```python
from build123d import *

# Parameters (mm, degrees)
SKETCH_1_W          = 26
SKETCH_1_H          = 16
EXTRUDE_1_DEPTH     = 2
EXTRUDE_2_DEPTH     = 2
FILLET_1_R          = 5
FILLET_2_R          = 3
SKETCH_4_R          = 4
CUT_EXTRUDE_1_DEPTH = 38.312866414
SKETCH_5_R          = 2.15
CUT_EXTRUDE_2_DEPTH = 34.648922717
FILLET_3_R          = 3
FILLET_START        = -13
FILLET_4_DEPTH      = 26.69955789
FILLET_START_2      = 4
FILLET_4_2_DEPTH    = 2


with BuildPart() as part:
    # 草图1 → 凸台-拉伸1 (new body)
    with BuildSketch(Plane(origin=(0, 0, 0), x_dir=(1, 0, 0), z_dir=(0, 1, 0))):
        Rectangle(SKETCH_1_W, SKETCH_1_H)
    extrude(amount=EXTRUDE_1_DEPTH)

    # 草图3 → 凸台-拉伸2 (add)
    with BuildSketch(Plane.XY.offset(8)):
        with BuildLine():
            Line((-13, 2), (-13, 8.5))
            Line((-13, 8.5), (0, 8.5))
            ThreePointArc((0, 8.5), (7.423811989, 10.173553708), (13.411524732, 14.870474248))
            ThreePointArc((13.411524732, 14.870474248), (28.449822139, 10.422228722), (14.725126476, 2.834738617))
            ThreePointArc((14.725126476, 2.834738617), (13.600854496, 2.958234042), (13, 2))
            Line((13, 2), (-13, 2))
        make_face()
    extrude(amount=-EXTRUDE_2_DEPTH)

    # 圆角1
    fillet_1_edges = [part.edges().sort_by_distance(p)[0] for p in [
        (-13, 8.5, 7),
    ]]
    fillet(fillet_1_edges, radius=FILLET_1_R)

    # 圆角2
    fillet_2_edges = [part.edges().sort_by_distance(p)[0] for p in [
        (-13, 1, -8),
        (13, 1, -8),
    ]]
    fillet(fillet_2_edges, radius=FILLET_2_R)

    # 草图4 → 切除-拉伸1 (cut, through all)
    with BuildSketch(Plane.XY.offset(8)):
        with Locations((20, 9.5)):
            Circle(SKETCH_4_R)
    extrude(amount=-CUT_EXTRUDE_1_DEPTH, mode=Mode.SUBTRACT)

    # 草图5 → 切除-拉伸2 (cut, through all)
    with BuildSketch(Plane(origin=(0, 2, 0), x_dir=(1, 0, 0), z_dir=(0, 1, 0))):
        with Locations(Location((-7, 1, 0), (0, 0, 270))):
            Circle(SKETCH_5_R)
        with Locations(Location((6, 1, 0), (0, 0, 270))):
            Circle(SKETCH_5_R)
    extrude(amount=-CUT_EXTRUDE_2_DEPTH, mode=Mode.SUBTRACT)

    # 圆角3
    fillet_3_edges = [part.edges().sort_by_distance(p)[0] for p in [
        (0, 0, 8),
    ]]
    fillet(fillet_3_edges, radius=FILLET_3_R)

    # 圆角4: read off the stored shape, not the designer's step
    # 圆角4 outline → 圆角4 (add)
    with BuildSketch(Plane.YZ.offset(FILLET_START)):
        with BuildLine():
            ThreePointArc((2, 5), (2.292893219, 5.707106781), (3, 6))
            Line((3, 6), (2, 6))
            Line((2, 6), (2, 5))
        make_face()
    extrude(amount=FILLET_4_DEPTH)

    # Fillet 4 2 outline → Fillet 4 2 (cut)
    with BuildSketch(Plane.XY.offset(FILLET_START_2)):
        with BuildLine():
            Line((13.69955789, 2), (13.699557878, 3.000000032))
            ThreePointArc((13.699557878, 3.000000032), (13.19224914, 2.610200695), (13, 1.999999133))
            Line((13, 1.999999133), (13.69955789, 2))
        make_face()
    extrude(amount=FILLET_4_2_DEPTH, mode=Mode.SUBTRACT)


solid = part.part
```
Work out the finished part from the listing and answer in its coordinate system (mm). A direction names the side the tool comes from. Coordinates: 2 decimals unless noted, no trailing zeros. Write each loop counter-clockwise with the first axis right and the second up, starting at its lowest first coordinate (ties: lowest second). Pieces come first, ordered by that corner, then holes.
Q1. Which of the six approach directions +Z, -Z, +X, -X, +Y, -Y give full straight-line access (tool end or side, diameter ignored) to faces 1 (the face through (-4, 8.5, 7)), 2 (the face through (0, 2, -2)), 3 (the face through (0, 0, -2))?
Q2. A cutting plane is placed at A-A, the plane x = -7. Give the vertices of the cut face in (y, z), then the cut area to 3 significant figures.
Q3. A cutting plane is placed at C-C, the plane x = 20. Give the vertices of the cut face in (y, z), then the cut area to 3 significant figures.
Q4. Find the intervals of material crossed by line 1 (X direction, y = 0.6, z = -1); line 2 (Y direction, x = -4, z = -5); line 3 (Z direction, x = 15.5, y = 3.75), in increasing order.
Q5. A cutting plane is placed at D-D, the plane z = 0.75. Give the vertices of the cut face in (x, y), then the cut area to 3 significant figures.
Q6. A cutting plane is placed at B-B, the plane y = 12.75. Give the vertices of the cut face in (x, z), then the cut area to 3 significant figures.
Q7. Determine the mould class of faces 4 (the face through (8.13, 1.01, -1.28)), 5 (the face through (0.54, 0.86, 7.1)), 6 (the face through (-4.87, 1.01, -1.28)), 7 (the face through (-11.57, 7, 6.99)) for opening direction Z: released by +Z, released by -Z, zero draft, split by the parting line, or undercut.
Q8. Each of these flat-tipped pins is pushed along its axis until it touches: pin 1 Ø5.5 at (x, z) = (-7, -1) entering from +Y; pin 2 Ø0.6 at (y, z) = (1, -1) entering from +X; pin 3 Ø1.5 at (x, z) = (-5, -3.5) entering from -Y; pin 4 Ø2 at (x, z) = (-2.5, 7) entering from +Y. Where does it stop, or does it pass through?
Findings below:
1. face 1: +Z, -Z, -X, +Y
1. face 2: -Z, +X, -X, +Y
1. face 3: +Z, -Z, +X, -X, -Y
2. outline: (0, -8) - (2, -8) - (2, -3.15) - (0, -3.15) - close; (0, 1.15) - (2, 1.15) - (2, 5) arc R1 cw to (3, 6) - (8.5, 6) - (8.5, 8) - (3, 8) arc R3 ccw to (0, 5) - close
2. area: 34.7 mm2
3. outline: (1, 6) - (5.5, 6) - (5.5, 8) - (1, 8) - close; (13.5, 6) - (18, 6) - (18, 8) - (13.5, 8) - close
3. area: 18.0 mm2
4. line 1: x = -13 to -9.15, -4.85 to 3.85, 8.15 to 13
4. line 2: y = 0 to 2
4. line 3: z = 6 to 8
5. outline: (-13, 0) - (-8.25, 0) - (-8.25, 2) - (-13, 2) - close; (-5.75, 0) - (4.75, 0) - (4.75, 2) - (-5.75, 2) - close; (7.25, 0) - (13, 0) - (13, 2) - (7.25, 2) - close
5. area: 42.0 mm2
6. outline: (11.36, 6) - (17.67, 6) - (17.67, 8) - (11.36, 8) - close; (22.33, 6) - (27.85, 6) - (27.85, 8) - (22.33, 8) - close
6. area: 23.7 mm2
7. face 4: undercut
7. face 5: released by +Z
7. face 6: undercut
7. face 7: zero draft
8. pin 1: stops at y = 2
8. pin 2: stops at x = 13
8. pin 3: stops at y = 0
8. pin 4: stops at y = 8.5
